Autodesk Fusion 360 part; units mm, degrees
sketch "Sketch1" plane through (0, 0, 0) normal (0, 0, 1) x (1, 0, 0)
  line L0 (0, 0) -> (115.84, 0)
  line L1 (115.84, 0) -> (115.84, 117)
  line L2 (115.84, 117) -> (0, 117)
  line L3 (0, 117) -> (0, 0)
  line L4 (10, 7) -> (105.84, 7)
  line L5 (105.84, 7) -> (105.84, 112)
  line L6 (105.84, 112) -> (10, 112)
  line L7 (10, 112) -> (10, 7)
  circle A0 centre (5, 112) radius 1.6
  circle A1 centre (5, 5) radius 1.6
  circle A2 centre (110.84, 5) radius 1.6
  circle A3 centre (110.84, 112) radius 1.6
  dimension "d1" = 115.84
  dimension "d2" = 117
  dimension "d3" = 95.84
  dimension "d4" = 105
  dimension "d6" = 10
  dimension "d7" = 5
  dimension "d8" = 3.2
  dimension "d9" = 5
  dimension "d10" = 5
  dimension "d11" = 3.2
  dimension "d12" = 5
  dimension "d13" = 5
  dimension "d14" = 3.2
  dimension "d15" = 5
  dimension "d16" = 5
  dimension "d17" = 3.2
  dimension "d18" = 5
  dimension "d19" = 5
extrude "Extrude1" add sketch "Sketch1" along normal blind 5 contours L0 L1 L2 L3 | L4 L5 L6 L7
fillet "Fillet1" radius 5 4 edges at (115.84, 117, 2.5) (115.84, 0, 2.5) (0, 117, 2.5) (0, 0, 2.5)
Could you check a few things on this model? Use its own coordinates, in mm. Give positions to 0.01 mm unless a question says otherwise; leave off trailing zeros.
Item 1: I'm going to push a flat-ended pin straight in: pin 1 (2.5 mm diameter, centred on x = 5, y = 112, fed in from -Z). Where does the tip first touch, or does it pass through?
Item 2: If we mould it in two halves opening along X, with no side actions, what happens to faces 1 (the face through (0, 59, 2)), 2 (the face through (114.34, 1.43, 2.54)), 3 (the face through (109.24, 4.93, 2.46))? For each: pulls with the +X half, pulls with the -X half, needs draft (parallel to the pull), parting line crosses it, or undercut.
Item 3: I need wall thicknesses on line 1 (Y direction, x = 110.84, z = 2.1); line 2 (X direction, y = 112, z = 4). Which ranges of each line are inside material? Lowest first, please.
Values:
1. pin 1: passes through
2. face 1: pulls with the -X half
2. face 2: pulls with the +X half
2. face 3: undercut
3. line 1: y = 0 to 3.4, 6.6 to 110.4, 113.6 to 117
3. line 2: x = 0 to 3.4, 6.6 to 109.24, 112.44 to 115.84
